For this review, use the dimensioned drawing (mm, ordinates from the lowest corner) and the shaded views. A direction names the side the tool comes from. Coordinates: 2 decimals unless noted, no trailing zeros. Loops run counter-clockwise (first coordinate to the right, second up) from the corner with the lowest first, then second, coordinate; pieces in that order, holes last.
1. To check wall thickness, follow probe 1 along X at (y, z) = (2.25, 2); probe 2 along Z at (x, y) = (11, 3.75); probe 3 along Y at (x, z) = (2.5, 2.25). State the ranges of each line that lie inside material, in increasing order.
2. Clearance check with flat-ended pins moving along their axes: P1, Ø3, axis at x = 10.5, z = 1.5, coming from the +Y side (1 decimal); P2, Ø2, axis at x = 5.5, z = 2.5, coming from the -Y side; P3, Ø1.5, axis at y = 6.5, z = 5, coming from the -X side. State where each tip first meets the part, or that it passes through.
3. Take a section at A-A, the plane y = 3.81. State the section outline as (x, z) points.
4. Machinability: for the marked faces 1 and 2, which of the approach directions +Z, -Z, +X, -X, +Y, -Y give a long, thin tool a straight path to every point of the face, cutting with its end or side? Answer none if there is none.
5. Take a section at B-B, the plane x = 1.5. State the section outline as (y, z) points.
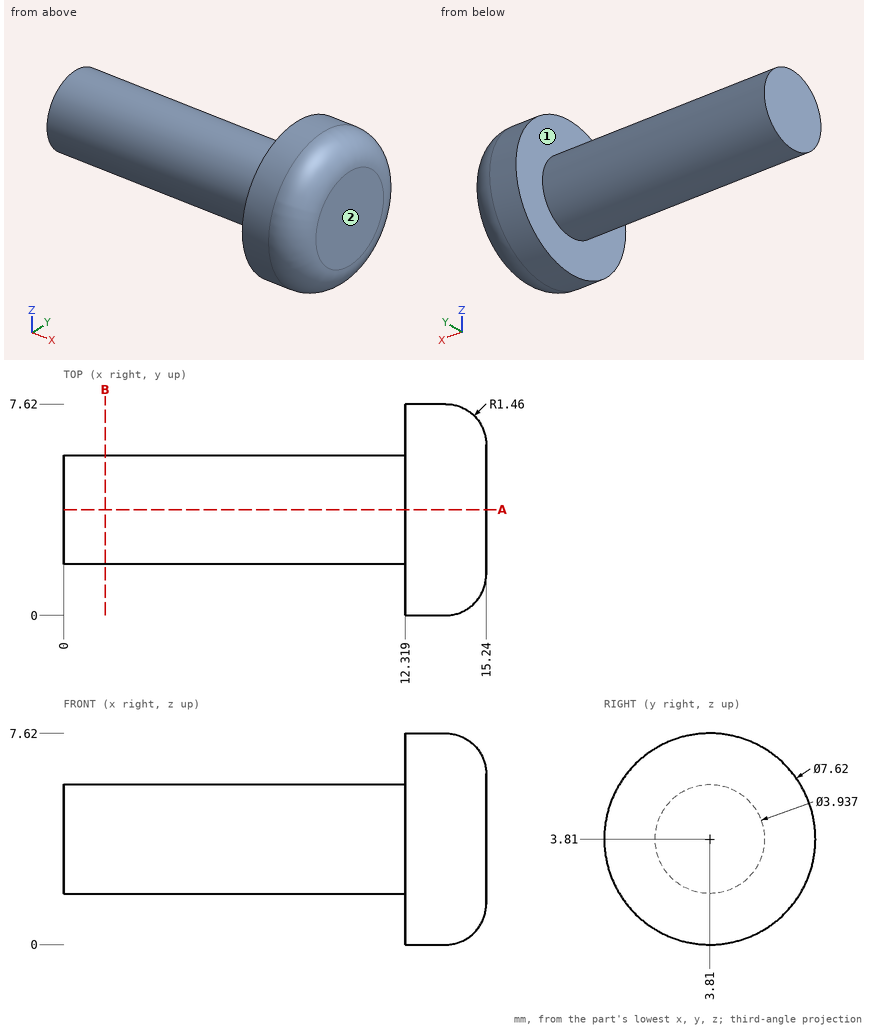
Results list:
1. probe 1: x = 12.32 to 15.24
1. probe 2: z = 1.84 to 5.78
1. probe 3: y = 2.61 to 5.01
2. P1: stops at y = 5.6
2. P2: stops at y = 1.87
2. P3: stops at x = 12.32
3. outline: (0, 1.84) - (12.32, 1.84) - (12.32, 0) - (13.78, 0) arc R1.46 ccw to (15.24, 1.46) - (15.24, 6.16) arc R1.46 ccw to (13.78, 7.62) - (12.32, 7.62) - (12.32, 5.78) - (0, 5.78) - close
4. face 1: -X
4. face 2: +Z, -Z, +X, +Y, -Y
5. outline: circle Ø3.94 at (3.81, 3.81)
